Geometry check sheet. Reference: the model listing, model coordinates, mm. A direction names the side the tool comes from. Give positions to 0.01 mm unless a question says otherwise; leave off trailing zeros. Order: outer loops, then holes, each group sorted by start corner. A loop starts at its lowest first (then second) coordinate and runs counter-clockwise, first axis right, second up. Notation, with made-up numbers: M 46.5,43.25 L 95.5,43.25 A26 cw 95.5,58.25 Z; hole C -29,16 d4. An arc over 180 degrees is marked long. Put each result on its own line as item: value. Start each with the question number.
Q1. Go/stop test with flat-tipped pins: pin 1 (1 mm diameter, centred on x = 5, y = -1.5, fed in from -Z); pin 2 (8.5 mm diameter, centred on y = -26.5, z = 17, fed in from +X) (3 decimals); pin 3 (6 mm diameter, centred on x = -0.5, z = 17.5, fed in from +Y). Record where each tip stops, or that it passes through.
Q2. Section check C-C on z = -5.5. Record the cut outline in (x, y), then the cut area to 3 significant figures.
Q3. Access from +Z, -Z, +X, -X, +Y, -Y to the whole of each face (thin tool, end or side, straight path). Record for faces 1 (the flat face through (0, -152.4, 0)), 2 (the flat face through (-4.445, -38, 16)), 3 (the flat face through (4.445, -38, 16)).
Q4. Section check A-A on x = 0. Record the cut outline in (y, z).
Q5. Section check D-D on y = 13. Record the cut outline in (x, z) (3 decimals).
Q6. Section check B-B on y = -14.5. Record the cut outline in (x, z) (3 decimals).
Q7. Material ranges on L1, parallel to X at y = -38.5, z = 18 (3 decimals); L2, parallel to X at y = -118, z = -1, recorded low to high.
```python
from build123d import *

# Parameters (mm, degrees)
F1_DEPTH      = 76.2
F2_DEPTH      = 76.2
F2_DEPTH_BACK = 152.4


with BuildPart() as f1:
    # F0 (on Front) → F1 (new body)
    with BuildSketch(Plane.XZ):
        with BuildLine():
            ThreePointArc((-4.445, 11.8967211869), (-7.2401139494, -10.4341147205), (12.7, 0))
            ThreePointArc((12.7, 0), (10.4341147205, 7.2401139494), (4.445, 11.8967211869))
            ThreePointArc((4.445, 11.8967211869), (0, 12.7), (-4.445, 11.8967211869))
        make_face()
        with BuildLine():
            ThreePointArc((-4.445, 11.8967211869), (0, 12.7), (4.445, 11.8967211869))
            Line((4.445, 11.8967211869), (4.445, 19.5167211869))
            Line((4.445, 19.5167211869), (-4.445, 19.5167211869))
            Line((-4.445, 19.5167211869), (-4.445, 11.8967211869))
        make_face()
    extrude(amount=F1_DEPTH)

    # F0 (on Front) → F2 (join, two sides)
    with BuildSketch(Plane.XZ) as f2_sk:
        with BuildLine():
            ThreePointArc((-4.445, 11.8967211869), (-7.2401139494, -10.4341147205), (12.7, 0))
            ThreePointArc((12.7, 0), (10.4341147205, 7.2401139494), (4.445, 11.8967211869))
            ThreePointArc((4.445, 11.8967211869), (0, 12.7), (-4.445, 11.8967211869))
        make_face()
    extrude(amount=-F2_DEPTH)
    extrude(f2_sk.sketch, amount=F2_DEPTH_BACK)


solid = f1.part
```
Results found:
1. pin 1: stops at z = -11.88
1. pin 2: stops at x = 4.445
1. pin 3: stops at y = 0
2. outline: M -11.45,-152.4 L 11.45,-152.4 L 11.45,76.2 L -11.45,76.2 Z
2. area: 5,230 mm^2
3. face 1: +Z, -Z, +X, -X, -Y
3. face 2: +Z, -X, +Y, -Y
3. face 3: +Z, +X, +Y, -Y
4. outline: M -152.4,-12.7 L 76.2,-12.7 L 76.2,12.7 L 0,12.7 L 0,19.52 L -76.2,19.52 L -76.2,12.7 L -152.4,12.7 Z
5. outline: C 0,0 d25.4
6. outline: M -4.445,11.897 A12.7 ccw long 4.445,11.897 L 4.445,19.517 L -4.445,19.517 Z
7. L1: x = -4.445 to 4.445
7. L2: x = -12.66 to 12.66
